Can you work these out from the drawing? Everything is in mm from the part's minimum corner. Coordinates: 2 decimals unless noted, no trailing zeros. Loops run counter-clockwise (first coordinate to the right, second up) from the corner with the lowest first, then second, coordinate; pieces in that order, holes last. Notation, with made-up numbers: M 36,22.5 L 81,22.5 A22 cw 81,28.5 Z; hole C 2.25,-13 d10. An arc over 180 degrees is marked long. Write each question's results on one line, items separated by ' | '.
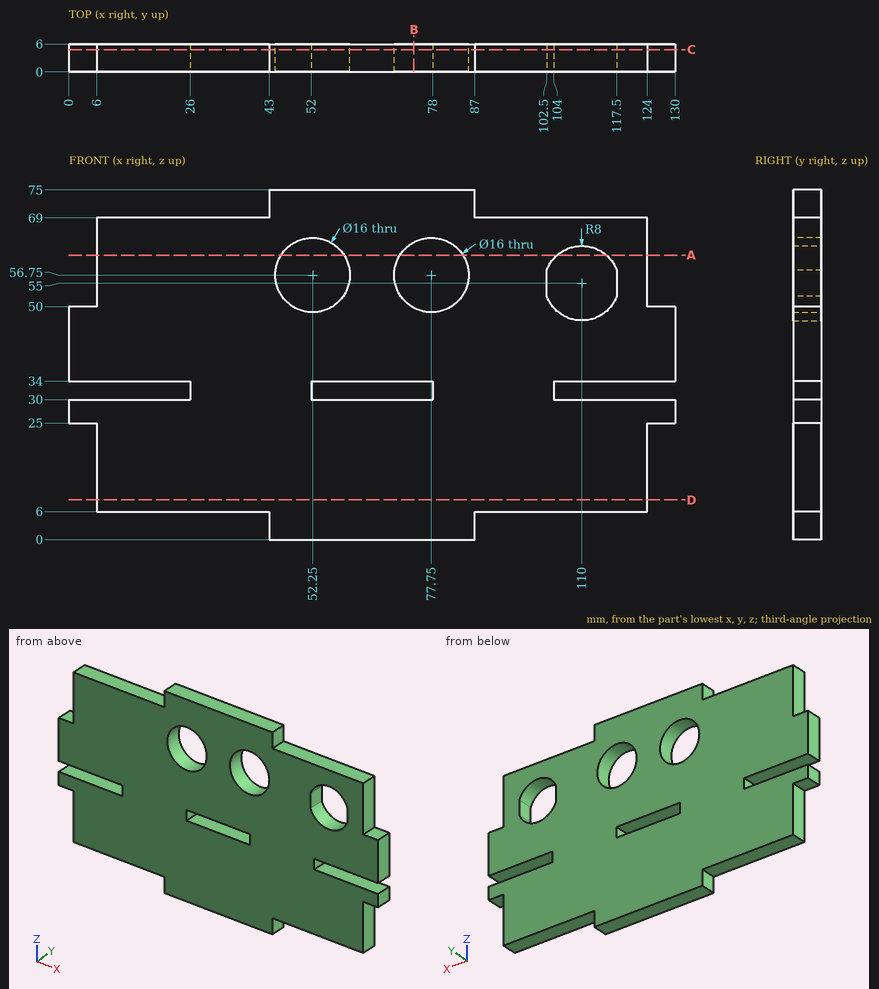
(1) Will these pins go through, and if not, where does the flat tip stop? P1, Ø1.8, axis at y = 3, z = 1.5, coming from the -X side; P2, Ø1.8, axis at y = 2, z = 11, coming from the +X side; P3, Ø2, axis at x = 103, y = 3.5, coming from the +Z side.
Reported:
P1: stops at x = 43 | P2: stops at x = 124 | P3: stops at z = 69
(2) Imagine slicing it at B-B, the plane x = 74. List the corners of the cut face in (y, z) for me.
Reported:
outline: M 0,0 L 6,0 L 6,30 L 0,30 Z; M 0,34 L 6,34 L 6,49.68 L 0,49.68 Z; M 0,63.82 L 6,63.82 L 6,75 L 0,75 Z
(3) Imagine slicing it at A-A, the plane z = 61. List the corners of the cut face in (x, y) for me, and give its area (3 significant figures).
Reported:
outline: M 6,0 L 45.47,0 L 45.47,6 L 6,6 Z; M 59.03,0 L 70.97,0 L 70.97,6 L 59.03,6 Z; M 84.53,0 L 104.71,0 L 104.71,6 L 84.53,6 Z; M 115.29,0 L 124,0 L 124,6 L 115.29,6 Z | area: 482 mm2
(4) Imagine slicing it at C-C, the plane y = 4.8. State how many separate pieces and enclosed holes the cut face has, and give its area (3 significant figures).
Reported:
separate pieces: 1 | enclosed holes: 4 | area: 7,350 mm2
(5) Please list where these lines run through material, in increasing order: probe 1 along X at (y, z) = (3.6, 56.75); probe 2 along Z at (x, y) = (67.5, 4.3); probe 3 along Z at (x, y) = (121, 0.7). Write a range as from..to.
Reported:
probe 1: x = 6..44.25, 60.25..69.75, 85.75..102.5, 117.5..124 | probe 2: z = 0..30, 34..75 | probe 3: z = 6..30, 34..69
(6) Imagine slicing it at D-D, the plane z = 8.5. List the corners of the cut face in (x, y) for me.
Reported:
outline: M 6,0 L 124,0 L 124,6 L 6,6 Z
